Work out the finished part from the listing and answer in its coordinate system (mm). A direction names the side the tool comes from. Give positions to 0.01 mm unless a question says otherwise; leave off trailing zeros. Order: outer loops, then holes, each group sorted by start corner. A loop starts at its lowest first (then second) coordinate and runs counter-clockwise, first axis right, second up. Notation, with made-up numbers: (33, -4) - (60, -4) arc R13 ccw to (60, 19) - close; hole circle Ø1 at (42.5, 57.5). An arc over 180 degrees is marked (long way). Write each question's results on one line, items separated by ' | '.
from build123d import *

# Parameters (mm, degrees)
F1_DEPTH  = 30
F2_W      = 90
F2_H      = 30
F3_DEPTH  = 15
F4_R      = 42.5
F5_DEPTH  = 5
F6_R      = 10
F7_DEPTH  = 5
F8_R      = 25
F9_DEPTH  = 5
F11_DEPTH = 20


with BuildPart() as f1:
    # F0 (on Top) → F1 (new body)
    with BuildSketch(Plane.XY):
        Polygon((82.968637, 80), (-82.968637, 80), (-78.04556, -80), (78.04556, -80), align=None)
        Polygon((-63.5, -65), (-67.5, 65), (67.5, 65), (63.5, -65), align=None, mode=Mode.SUBTRACT)
    extrude(amount=F1_DEPTH)

    # F2 (on face) → F3 (cut, through all)
    with BuildSketch(Plane.XZ.offset(80)):
        with Locations((0, 15)):
            Rectangle(F2_W, F2_H)
    extrude(amount=-F3_DEPTH, mode=Mode.SUBTRACT)

    # F4 (on Top) → F5 (join)
    with BuildSketch(Plane.XY):
        Polygon((82.968637, 80), (-82.968637, 80), (-78.04556, -80), (-45, -80), (-45, -65), (45, -65), (45, -80), (78.04556, -80), align=None)
        Circle(F4_R, mode=Mode.SUBTRACT)
    extrude(amount=-F5_DEPTH)

    # F8 (on face) → F9 (join)
    with BuildSketch(Plane(origin=(0, 0, -5), x_dir=(1, 0, 0), z_dir=(0, 0, -1))):
        Polygon((-45, 80), (-78.04556, 80), (-82.968637, -80), (82.968637, -80), (78.04556, 80), (45, 80), (45, 65), (-45, 65), align=None)
        Circle(F8_R, mode=Mode.SUBTRACT)
    extrude(amount=F9_DEPTH)



with BuildPart() as f7:
    # F6 (on face) → F7 (new body)
    with BuildSketch(Plane(origin=(0, 0, -5), x_dir=(1, 0, 0), z_dir=(0, 0, -1))):
        Circle(F6_R)
    extrude(amount=F7_DEPTH)


with BuildPart() as f1_1:
    add(f1.part)

    add(f7.part)  # F11 merges F7
    # F10 (on face) → F11 (join)
    with BuildSketch(Plane(origin=(0, 0, -10), x_dir=(1, 0, 0), z_dir=(0, 0, -1))):
        Polygon((-78.04556, 80), (-82.968637, -80), (82.968637, -80), (78.04556, 80), (45, 80), (45, 65), (-45, 65), (-45, 80), align=None)
    extrude(amount=F11_DEPTH)


solid = f1_1.part
1. A cutting plane is placed at C-C, the plane z = -24.5. Write down the section's boundary in (x, y).
Answer list:
outline: (-82.97, 80) - (-78.05, -80) - (-45, -80) - (-45, -65) - (45, -65) - (45, -80) - (78.05, -80) - (82.97, 80) - close
2. Straight lines are drawn through the part: line 1 (Y direction, x = 0, z = -6.85); line 2 (X direction, y = 0, z = -6.05); line 3 (Y direction, x = -2.5, z = -8.5). For each, find the intervals that lie inside material, in ascending order. Write a range as [from, to].
Answer list:
line 1: [-65, -25], [-10, 10], [25, 80] | line 2: [-80.51, -25], [-10, 10], [25, 80.51] | line 3: [-65, -24.87], [-9.68, 9.68], [24.87, 80]
3. A tool of negligible diameter and unlimited length cuts with its end or side. For faces 4 (the face through (-61, -80, 0)), 5 (the face through (-45, -72, 0)), 6 (the face through (-54, -65, 15)), from which of +Z, -Z, +X, -X, +Y, -Y can it reach the whole face along a straight path? Write none if from no direction.
Answer list:
face 4: +Z, -Z, +X, -X, -Y | face 5: +Z, -Z, -Y | face 6: +Z
4. A cutting plane is placed at D-D, the plane y = 0. Write down the section's boundary in (x, z).
Answer list:
outline: (-80.51, -30) - (80.51, -30) - (80.51, 30) - (65.5, 30) - (65.5, 0) - (42.5, 0) - (42.5, -5) - (25, -5) - (25, -10) - (10, -10) - (10, -5) - (-10, -5) - (-10, -10) - (-25, -10) - (-25, -5) - (-42.5, -5) - (-42.5, 0) - (-65.5, 0) - (-65.5, 30) - (-80.51, 30) - close
5. A cutting plane is placed at A-A, the plane z = -8. Write down the section's boundary in (x, y), then the cut area to 3 significant figures.
Answer list:
outline: (-82.97, 80) - (-78.05, -80) - (-45, -80) - (-45, -65) - (45, -65) - (45, -80) - (78.05, -80) - (82.97, 80) - close; circle Ø20 at (0, 0); hole circle Ø50 at (0, 0) | area: 22,800 mm^2
6. Given P1, Ø5, axis at y = -57, z = 10, coming from the +X side; P2, Ø4, axis at y = 37.5, z = -16, coming from the -X side; P3, Ø15, axis at x = -14.5, z = -18, coming from the -Y side, each flat-ended and moving along its own axis, determine where each tip first touches the part or whether it passes through.
Answer list:
P1: x = 78.83 | P2: x = -81.72 | P3: y = -65
7. Determine the mould class of faces 1 (the face through (-31, 30, 0)), 2 (the face through (-33.727, -25.861, -2.465)), 3 (the face through (62, -80, 0)) for opening direction X: +X half, -X half, draft (parallel to the pull), parting line (faces both ways), or undercut.
Answer list:
face 1: undercut | face 2: undercut | face 3: draft
8. A cutting plane is placed at B-B, the plane x = 0. Write down the section's boundary in (y, z), then the cut area to 4 significant figures.
Answer list:
outline: (-65, -30) - (80, -30) - (80, 30) - (65, 30) - (65, 0) - (42.5, 0) - (42.5, -5) - (25, -5) - (25, -10) - (10, -10) - (10, -5) - (-10, -5) - (-10, -10) - (-25, -10) - (-25, -5) - (-42.5, -5) - (-42.5, 0) - (-65, 0) - close | area: 4,225 mm^2
